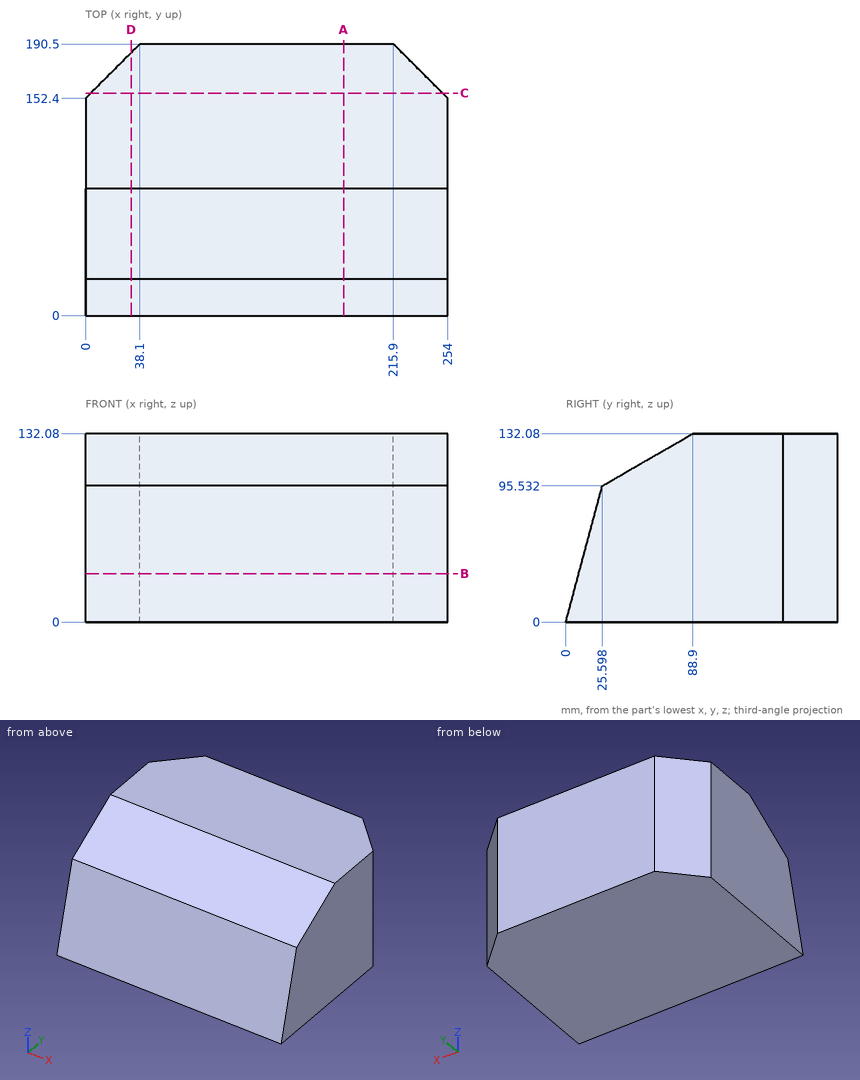
The figure shows three views and two pictorial views of one solid part (mm, origin at its lowest corner). Answer the questions. Round coordinates to 2 decimals unless told otherwise and drop trailing zeros. Order: outer loops, then holes, each group sorted by start corner. A loop starts at its lowest first (then second) coordinate and runs counter-clockwise, first axis right, second up. Notation, with made-up numbers: (63, 29.5) -> (98, 29.5) arc R10 ccw to (98, 47.5) -> close; hole circle Ø8 at (-20.5, 86.5). An arc over 180 degrees is marked (long way). One line per item, written item: value.
Item 1: Find section C-C, the plane y = 156. Give the vertices of the cut face in (x, z), then the cut area to 3 significant figures.
Taken from the geometry:
outline: (3.6, 0) -> (250.4, 0) -> (250.4, 132.08) -> (3.6, 132.08) -> close
area: 32,600 mm2
Item 2: Given P1, Ø3, axis at x = 29, z = 81, coming from the -Y side; P2, Ø1, axis at x = 95, z = 87.5, coming from the -Y side; P3, Ø1.5, axis at x = 26, z = 80, coming from the -Y side (1 decimal), each flat-ended and moving along its own axis, determine where each tip first touches the part or whether it passes through.
Taken from the geometry:
P1: stops at y = 21.3
P2: stops at y = 23.31
P3: stops at y = 21.2
Item 3: Find section A-A, the plane x = 181. Give the vertices of the cut face in (y, z), then the cut area to 3 significant figures.
Taken from the geometry:
outline: (0, 0) -> (190.5, 0) -> (190.5, 132.08) -> (88.9, 132.08) -> (25.6, 95.53) -> close
area: 21,800 mm2
Item 4: Find section D-D, the plane x = 32. Give the vertices of the cut face in (y, z).
Taken from the geometry:
outline: (0, 0) -> (184.4, 0) -> (184.4, 132.08) -> (88.9, 132.08) -> (25.6, 95.53) -> close
Item 5: Straight lines are drawn through the part: L1, parallel to Y at x = 111.5, z = 43.5 (1 decimal); L2, parallel to Y at x = 211, z = 10.5; L3, parallel to Z at x = 22.5, y = 35. For each, find the intervals that lie inside material, in ascending order.
Taken from the geometry:
L1: y = 11.7 to 190.5
L2: y = 2.81 to 190.5
L3: z = 0 to 100.96
Item 6: Find section B-B, the plane z = 34. Give the vertices of the cut face in (x, y).
Taken from the geometry:
outline: (0, 9.11) -> (254, 9.11) -> (254, 152.4) -> (215.9, 190.5) -> (38.1, 190.5) -> (0, 152.4) -> close
